Print and shaded views of the part. All mm, measured from the part's lowest x, y and z. A direction names the side the tool comes from. Coordinates: 2 decimals unless noted, no trailing zeros. Loops run counter-clockwise (first coordinate to the right, second up) from the corner with the lowest first, then second, coordinate; pieces in that order, holes last. Notation, with made-up numbers: (9, 44.25) -> (48, 44.25) arc R13 ccw to (48, 50.25) -> close; hole circle Ø10 at (73.25, 63). An arc over 180 degrees is marked (long way). One line per question, with ' | ' between items. Start each with the question number.
1) Probe L1, parallel to Y at x = 16, z = 7.5; L2, parallel to Y at x = 26.5, z = 4.75; L3, parallel to X at y = 35, z = 12 (1 decimal). List the from-to ranges inside material, lowest first. Write a range as from..to.
2) Drop flat-ended pins along their axis: pin 1 (7.5 mm diameter, centred on y = 23.5, z = 11.5, fed in from +X); pin 2 (8 mm diameter, centred on x = 32.5, y = 10, fed in from -Z); pin 3 (11 mm diameter, centred on y = 50.5, z = 13, fed in from -X); pin 4 (1 mm diameter, centred on x = 7, z = 22, fed in from +Y). Give the stop position or say it passes through.
3) Cut at B-B (z = 8.75). List the corners of the cut face in (x, y) (1 decimal), plus the area to 3 significant figures.
4) 3-axis set-ups, long thin cutter, end or side, ignore diameter. For the marked faces 1, 2, 3 and 4: which of +Z, -Z, +X, -X, +Y, -Y reach the whole face in a straight line?
5) Two-plate mould, pull along Y, no slides. Class the marked faces 5, 6 and 7: released by +Y, released by -Y, zero draft, split by the parting line, or undercut.
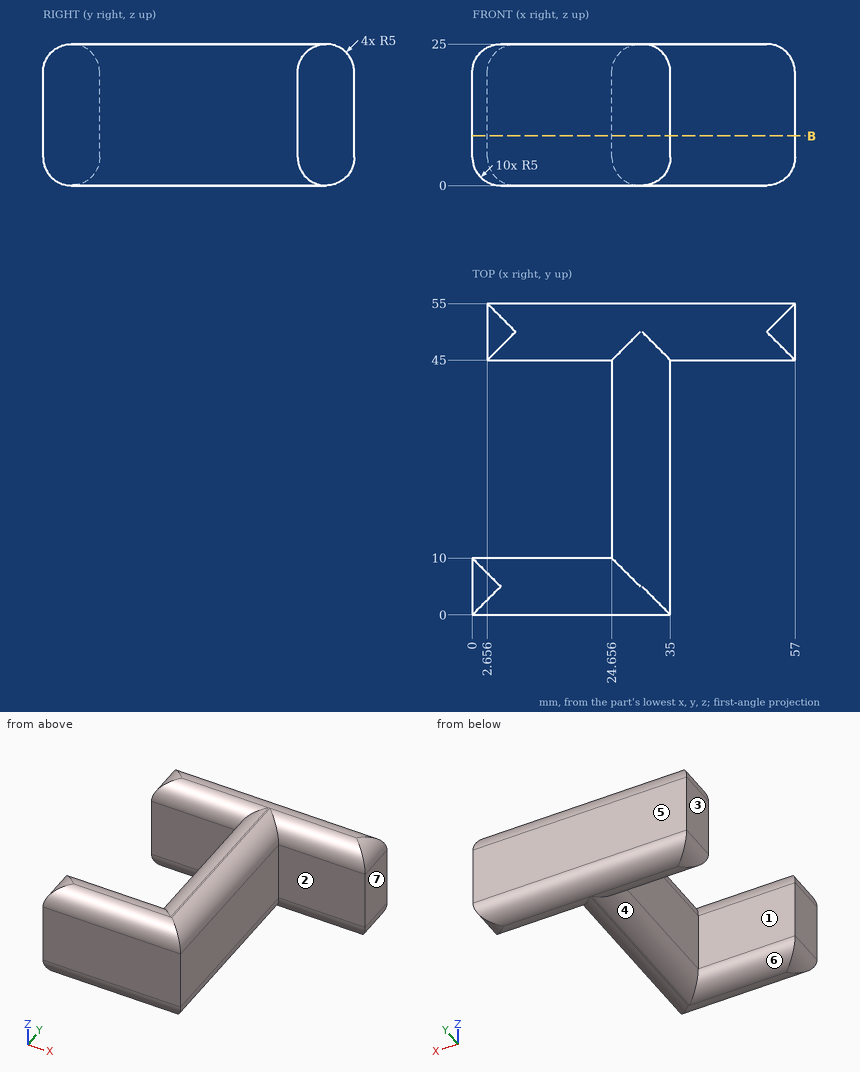
Reported:
1) L1: y = 0..10, 45..55 | L2: y = 0.01..54.99 | L3: x = 24.7..35
2) pin 1: stops at x = 35 | pin 2: stops at z = 0 | pin 3: stops at x = 2.66 | pin 4: stops at y = 54.77
3) outline: (0, 0) -> (35, 0) -> (35, 45) -> (57, 45) -> (57, 55) -> (2.7, 55) -> (2.7, 45) -> (24.7, 45) -> (24.7, 10) -> (0, 10) -> close | area: 1,260 mm²
4) face 1: +Z, -Z, -X | face 2: +Z, -Z, +X, -Y | face 3: +Z, -Z, -X, +Y | face 4: -Z, -X
5) face 5: released by +Y | face 6: undercut | face 7: zero draft
